```python
from build123d import *

# Parameters (mm, degrees)
ESQUISSE1_R                  = 11
ESQUISSE1_R_2                = 4.5
BOSS_EXTRU_1_DEPTH           = 4
ESQUISSE4_R                  = 11
BOSS_EXTRU_2_DEPTH           = 1
ESQUISSE2_R                  = 1.5
ENL_V_MAT_EXTRU_1_DEPTH      = 1
ENL_V_MAT_EXTRU_1_DEPTH_BACK = 6
ESQUISSE5_W                  = 6
ESQUISSE5_H                  = 6
BOSS_EXTRU_3_DEPTH           = 21
CHANFREIN1_SIZE              = 1
ESQUISSE8_R                  = 3.95
BOSS_EXTRU_4_DEPTH           = 12.5
ESQUISSE6_R                  = 1.75
ENL_V_MAT_EXTRU_2_DEPTH      = 1
ENL_V_MAT_EXTRU_2_DEPTH_BACK = 27


with BuildPart() as part:
    # Esquisse1 → Boss.-Extru.1 (new body)
    with BuildSketch(Plane.XY):
        Circle(ESQUISSE1_R)
        Circle(ESQUISSE1_R_2, mode=Mode.SUBTRACT)
    extrude(amount=BOSS_EXTRU_1_DEPTH)

    # Esquisse4 → Boss.-Extru.2 (add)
    with BuildSketch(Plane.XY.offset(4)):
        Circle(ESQUISSE4_R)
    extrude(amount=BOSS_EXTRU_2_DEPTH)

    # Esquisse2 → Enlèv. mat.-Extru.1 (cut, two sides)
    with BuildSketch(Plane.XY.offset(5)) as enl_v_mat_extru_1_sk:
        with Locations((8, 0)):
            Circle(ESQUISSE2_R)
        with Locations((5.656854249, -5.656854249)):
            Circle(ESQUISSE2_R)
        with Locations((0, -8)):
            Circle(ESQUISSE2_R)
        with Locations((-5.656854249, -5.656854249)):
            Circle(ESQUISSE2_R)
        with Locations((-8, 0)):
            Circle(ESQUISSE2_R)
        with Locations((-5.656854249, 5.656854249)):
            Circle(ESQUISSE2_R)
        with Locations((0, 8)):
            Circle(ESQUISSE2_R)
        with Locations((5.656854249, 5.656854249)):
            Circle(ESQUISSE2_R)
    extrude(amount=ENL_V_MAT_EXTRU_1_DEPTH, mode=Mode.SUBTRACT)
    extrude(enl_v_mat_extru_1_sk.sketch, amount=-ENL_V_MAT_EXTRU_1_DEPTH_BACK, mode=Mode.SUBTRACT)

    # Esquisse5 → Boss.-Extru.3 (add)
    with BuildSketch(Plane.XY.offset(5)):
        Rectangle(ESQUISSE5_W, ESQUISSE5_H)
    extrude(amount=BOSS_EXTRU_3_DEPTH)

    # Chanfrein1
    chanfrein1_edges = [part.edges().sort_by_distance(p)[0] for p in [
        (-3, 3, 15.5),
        (-3, -3, 15.5),
        (3, -3, 15.5),
        (3, 3, 15.5),
    ]]
    chamfer(chanfrein1_edges, length=CHANFREIN1_SIZE)

    # Esquisse8 → Boss.-Extru.4 (add)
    with BuildSketch(Plane.XY.offset(5)):
        Circle(ESQUISSE8_R)
    extrude(amount=BOSS_EXTRU_4_DEPTH)

    # Esquisse6 → Enlèv. mat.-Extru.2 (cut, two sides)
    with BuildSketch(Plane.XY.offset(26)) as enl_v_mat_extru_2_sk:
        Circle(ESQUISSE6_R)
    extrude(amount=ENL_V_MAT_EXTRU_2_DEPTH, mode=Mode.SUBTRACT)
    extrude(enl_v_mat_extru_2_sk.sketch, amount=-ENL_V_MAT_EXTRU_2_DEPTH_BACK, mode=Mode.SUBTRACT)


solid = part.part
```
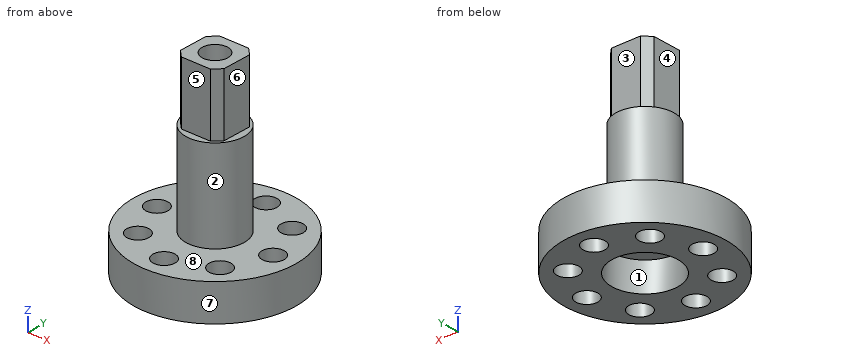
Design review of the part built by this model. Coordinates are the model's own, in mm. Face numbers are marked on the shaded views. A direction names the side the tool comes from. Give positions to 0.01 mm unless a question says otherwise; leave off trailing zeros. Loops run counter-clockwise (first coordinate to the right, second up) from the corner with the lowest first, then second, coordinate; pieces in that order, holes last. Notation, with made-up numbers: M 45,-9.75 L 75,-9.75 A24 cw 75,9.25 Z; hole C 54.25,34.5 d8. An arc over 180 degrees is marked long. Return JSON: item names as keys, results as strings. Group by question number.
Item 1: Tool access review of the marked faces 4, 5, 6, 7 and 8: name each direction out of +Z, -Z, +X, -X, +Y, -Y from which nothing blocks a thin tool from reaching the whole face with its end or side.
Item 2: We need section A-A (x = 0). Give the boundary of the cut face in (y, z), and give its area (3 significant figures).
Item 3: Mouldability with a two-part tool opening along X and no side actions: class the marked faces 1, 2 and 3 as released by +X, released by -X, zero draft, split by the parting line, or undercut.
Item 4: Insertion check: pin 1 Ø2.5 at (x, y) = (0, 8) entering from +Z; pin 2 Ø3 at (y, z) = (0, 22.5) entering from +X; pin 3 Ø2 at (x, z) = (-0.5, 23) entering from -Y; pin 4 Ø4.5 at (x, z) = (-0.5, 21.5) entering from +Y. Each pin has a flat end and moves straight along its axis. Give the tip position at first contact, or say it passes through.
Item 5: For probe 1 along Y at (x, z) = (0, 2.65); probe 2 along Z at (x, y) = (1.5, -9); probe 3 along Y at (x, z) = (0, 24.75), list the stretches that pass through material, from the lowest coordinate up.
Item 6: We need section D-D (x = 8). Give the boundary of the cut face in (y, z).
Item 7: We need section C-C (z = 23.5). Give the boundary of the cut face in (x, y), and give its area (3 significant figures).
Item 8: We need section B-B (y = -5.25). Give the boundary of the cut face in (x, z), and give its area (3 significant figures).
Output:
{
 "1": {"face 4": "+Z, -X, +Y, -Y", "face 5": "+Z, +X, -X, -Y", "face 6": "+Z, +X, +Y, -Y", "face 7": "+Z, -Z", "face 8": "+Z"},
 "2": {"outline": "M -11,0 L -9.5,0 L -9.5,5 L -11,5 Z; M -6.5,0 L -4.5,0 L -4.5,4 L -1.75,4 L -1.75,26 L -3,26 L -3,17.5 L -3.95,17.5 L -3.95,5 L -6.5,5 Z; M 1.75,4 L 4.5,4 L 4.5,0 L 6.5,0 L 6.5,5 L 3.95,5 L 3.95,17.5 L 3,17.5 L 3,26 L 1.75,26 Z; M 9.5,0 L 11,0 L 11,5 L 9.5,5 Z", "area": "117 mm^2"},
 "3": {"face 1": "undercut", "face 2": "split by the parting line", "face 3": "zero draft"},
 "4": {"pin 1": "passes through", "pin 2": "stops at x = 3", "pin 3": "stops at y = -3", "pin 4": "stops at y = 3"},
 "5": {"probe 1": "y = -11 to -9.5, -6.5 to -4.5, 4.5 to 6.5, 9.5 to 11", "probe 2": "z = 0 to 5", "probe 3": "y = -3 to -1.75, 1.75 to 3"},
 "6": {"outline": "M -7.55,0 L -1.5,0 L -1.5,5 L -7.55,5 Z; M 1.5,0 L 7.55,0 L 7.55,5 L 1.5,5 Z"},
 "7": {"outline": "M -3,-2 L -2,-3 L 2,-3 L 3,-2 L 3,2 L 2,3 L -2,3 L -3,2 Z; hole C 0,0 d3.5", "area": "24.4 mm^2"},
 "8": {"outline": "M -9.67,0 L -7.1,0 L -7.1,5 L -9.67,5 Z; M -4.21,0 L 4.21,0 L 4.21,5 L -4.21,5 Z; M 7.1,0 L 9.67,0 L 9.67,5 L 7.1,5 Z", "area": "67.8 mm^2"}
}
